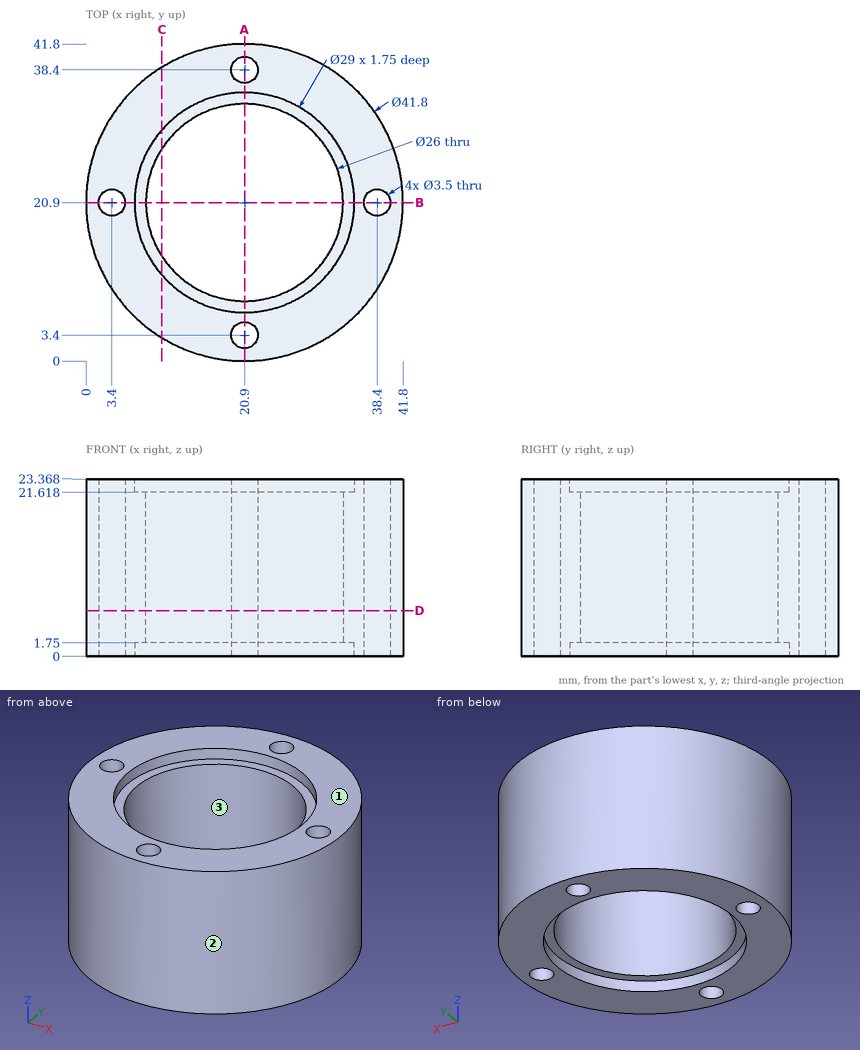
Study the drawing (mm; zero at the part's minimum x, y, z) and answer. Round coordinates to 2 decimals unless told otherwise and drop trailing zeros. Write each loop counter-clockwise with the first axis right and the second up, starting at its lowest first coordinate (ties: lowest second). Pieces come first, ordered by that corner, then holes.
Q1. The mould has two halves that part along X. Classify the marked faces 1, 2 and 3: released by +X, released by -X, zero draft, split by the parting line, or undercut.
Values:
face 1: zero draft
face 2: split by the parting line
face 3: undercut
Q2. Find section C-C on x = 10. Determine the outline of the cut face in (y, z).
Values:
outline: (3.07, 0) - (11.34, 0) - (11.34, 1.75) - (13.82, 1.75) - (13.82, 21.62) - (11.34, 21.62) - (11.34, 23.37) - (3.07, 23.37) - close; (27.98, 1.75) - (30.46, 1.75) - (30.46, 0) - (38.73, 0) - (38.73, 23.37) - (30.46, 23.37) - (30.46, 21.62) - (27.98, 21.62) - close
Q3. Find section A-A on x = 20.9. Determine the outline of the cut face in (y, z), and give its area (3 significant figures).
Values:
outline: (0, 0) - (1.65, 0) - (1.65, 23.37) - (0, 23.37) - close; (5.15, 0) - (6.4, 0) - (6.4, 1.75) - (7.9, 1.75) - (7.9, 21.62) - (6.4, 21.62) - (6.4, 23.37) - (5.15, 23.37) - close; (33.9, 1.75) - (35.4, 1.75) - (35.4, 0) - (36.65, 0) - (36.65, 23.37) - (35.4, 23.37) - (35.4, 21.62) - (33.9, 21.62) - close; (40.15, 0) - (41.8, 0) - (41.8, 23.37) - (40.15, 23.37) - close
area: 195 mm2
Q4. Straight lines are drawn through the part: line 1 (Y direction, x = 28.5, z = 12.25); line 2 (Y direction, x = 19.5, z = 2.5); line 3 (Y direction, x = 27, z = 16). For each, find the intervals that lie inside material, in ascending order.
Values:
line 1: y = 1.43 to 10.35, 31.45 to 40.37
line 2: y = 0.05 to 2.35, 4.45 to 7.98, 33.82 to 37.35, 39.45 to 41.75
line 3: y = 0.91 to 9.42, 32.38 to 40.89
Q5. Find section D-D on z = 6. Determine the outline of the cut face in (x, y).
Values:
outline: circle Ø41.8 at (20.9, 20.9); hole circle Ø3.5 at (3.4, 20.9); hole circle Ø26 at (20.9, 20.9); hole circle Ø3.5 at (20.9, 3.4); hole circle Ø3.5 at (20.9, 38.4); hole circle Ø3.5 at (38.4, 20.9)
Q6. Flat-ended cylindrical pins translate along their axes: P1, Ø8.5, axis at x = 16.5, y = 24.5, coming from the -Z side; P2, Ø3, axis at y = 13, z = 4.5, coming from the -X side; P3, Ø1.5, axis at x = 30, z = 4.5, coming from the -Y side; P4, Ø2, axis at x = 30, z = 18.5, coming from the +Y side. Find the tip coordinate at first contact, or state that the pin passes through.
Values:
P1: passes through
P2: stops at x = 1
P3: stops at y = 1.74
P4: stops at y = 40.17
